Read the model definition and answer for the solid it produces. Units are mm, in the model's axes. Face numbers are marked on the shaded views. A direction names the side the tool comes from. Give positions to 0.01 mm unless a question says otherwise; leave off trailing zeros. Write each loop counter-clockwise with the first axis right and the second up, starting at its lowest first coordinate (ties: lowest second). Pieces come first, ordered by that corner, then holes. Notation, with made-up numbers: M 73.5,-5 L 103.5,-5 A22 ccw 103.5,1 Z; hole C -34,-35.5 d5. An arc over 180 degrees is marked long. Use a Markdown table: item, result. Add a question column.
Item 1: For the marked faces 1 and 2, determine the directions among +Z, -Z, +X, -X, +Y, -Y from which every point of the face is accessible in a straight line to the end or side of a thin tool.
Item 2: A cutting plane is placed at A-A on z = 8. Count the separate pieces of the cut face and the enclosed holes in it, then the cut area to 3 significant figures.
Item 3: The mould has two halves that part along Y. Classify the marked faces 3, 4, 5 and 6: pulls with the +Y half, pulls with the -Y half, needs draft (parallel to the pull), parting line crosses it, or undercut.
Item 4: Consider probe 1 along Y at (x, z) = (12.5, 10.75); probe 2 along Y at (x, z) = (12.5, 1.8); probe 3 along X at (y, z) = (-5.5, 6.25). Determine where each line is inside the solid, lowest interval first. Write a range as [from, to].
Item 5: Given P1, Ø1.5, axis at y = 4, z = 9.5, coming from the -X side; P2, Ø7, axis at x = 12.5, y = 0, coming from the +Z side; P3, Ø2, axis at y = -3, z = 1.5, coming from the -X side, each flat-ended and moving along its own axis, determine where each tip first touches the part or whether it passes through.
Item 6: A cutting plane is placed at C-C on x = -11.5. Determine the outline of the cut face in (y, z), then the cut area to 3 significant figures.
from build123d import *

# Parameters (mm, degrees)
SKETCH2_W                               = 45
SKETCH2_H                               = 20
BOSS_EXTRUDE2_DEPTH                     = 14.16787265
FILLET1_R                               = 10
CUT_EXTRUDE1_DEPTH                      = 22
CBORE_FOR_M5_HEX_HEAD_BOLT1_D           = 5.5
CBORE_FOR_M5_HEX_HEAD_BOLT1_CBORE_D     = 12
CBORE_FOR_M5_HEX_HEAD_BOLT1_CBORE_DEPTH = 10
FILLET2_R                               = 3


with BuildPart() as part:
    # Sketch2 → Boss-Extrude2 (new body)
    with BuildSketch(Plane.XY):
        Rectangle(SKETCH2_W, SKETCH2_H)
    extrude(amount=BOSS_EXTRUDE2_DEPTH)

    # Fillet1
    fillet1_edges = [part.edges().sort_by_distance(p)[0] for p in [
        (22.5, 10, 7.083936325),
        (22.5, -10, 7.083936325),
        (-22.5, 10, 7.083936325),
        (-22.5, -10, 7.083936325),
    ]]
    fillet(fillet1_edges, radius=FILLET1_R - 0.0001)  # a hair under: the kernel refuses the full size

    # Sketch3 → Cut-Extrude1 (cut)
    with BuildSketch(Plane.XZ.offset(10)):
        with BuildLine():
            Line((-5, 0), (-5, 4))
            ThreePointArc((-5, 4), (0, 9), (5, 4))
            Line((5, 4), (5, 0))
            ThreePointArc((5, 0), (0, -5), (-5, 0))
        make_face()
    extrude(amount=-CUT_EXTRUDE1_DEPTH, mode=Mode.SUBTRACT)

    # CBORE for M5 Hex Head Bolt1 (through all)
    with Locations(Plane.XY.offset(14.16787265)):
        with Locations((-12.5, 0), (12.5, 0)):
            CounterBoreHole(CBORE_FOR_M5_HEX_HEAD_BOLT1_D / 2, CBORE_FOR_M5_HEX_HEAD_BOLT1_CBORE_D / 2, CBORE_FOR_M5_HEX_HEAD_BOLT1_CBORE_DEPTH)

    # Fillet2
    fillet2_edges = [part.edges().sort_by_distance(p)[0] for p in [
        (0, 10, 14.16787265),
        (0, -10, 14.16787265),
        (-19.571097101, -7.071097101, 14.16787265),
        (-19.571097101, 7.071097101, 14.16787265),
        (19.571097101, -7.071097101, 14.16787265),
        (19.571097101, 7.071097101, 14.16787265),
    ]]
    fillet(fillet2_edges, radius=FILLET2_R)


solid = part.part
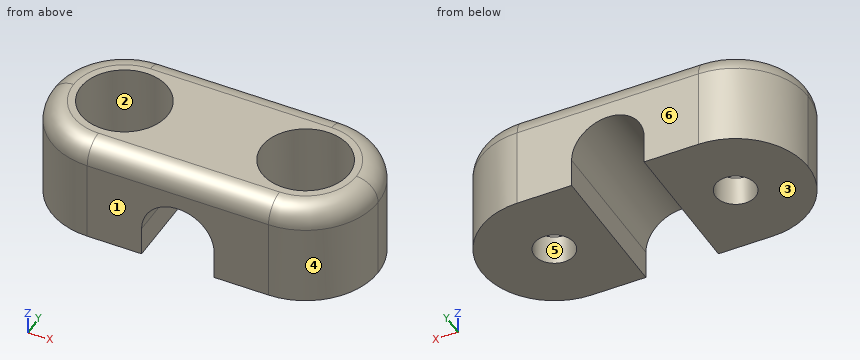
Filled in:
| question | item | result |
|---|---|---|
| 1 | face 1 | +Z, -Z, +X, -X, -Y |
| 1 | face 2 | +Z |
| 2 | separate pieces | 2 |
| 2 | enclosed holes | 2 |
| 2 | area | 468 mm² |
| 3 | face 3 | needs draft |
| 3 | face 4 | pulls with the -Y half |
| 3 | face 5 | undercut |
| 3 | face 6 | pulls with the +Y half |
| 4 | probe 1 | [-10, -6], [6, 10] |
| 4 | probe 2 | [-10, -2.75], [2.75, 10] |
| 4 | probe 3 | [-20.85, -14.9], [-10.1, -4.47], [4.47, 10.1], [14.9, 20.85] |
| 5 | P1 | x = -21.96 |
| 5 | P2 | z = 4.17 |
| 5 | P3 | x = -22.3 |
| 6 | outline | M -10,0 L -2.56,0 L -2.56,4.17 L -5.92,4.17 L -5.92,14.17 L -7,14.17 A3 ccw -10,11.17 Z; M 2.56,0 L 10,0 L 10,11.17 A3 ccw 7,14.17 L 5.92,14.17 L 5.92,4.17 L 2.56,4.17 Z |
| 6 | area | 140 mm² |
